Here's how the part is built. I have some questions about the finished solid (model axes, mm). Face numbers are marked on the shaded views. A direction names the side the tool comes from. Round coordinates to 2 decimals unless told otherwise and drop trailing zeros. Order: outer loops, then holes, each group sorted by start corner. A loop starts at its lowest first (then second) coordinate and runs counter-clockwise, first axis right, second up. Notation, with made-up numbers: (5.25, 36.5) - (45.25, 36.5) arc R32 ccw to (45.25, 63.5) - close; hole circle Ø8 at (13, 60). An arc over 180 degrees is marked (long way). Answer as a JSON object with one key per item and string values.
```python
from build123d import *

# Parameters (mm, degrees)
F0_R      = 14.5
F1_DEPTH  = 2
F2_R      = 11
F3_DEPTH  = 20
F4_R      = 2.075
F5_DEPTH  = 22.001
F6_W      = 3
F6_H      = 3.4
F7_DEPTH  = 2
F8_R      = 0.8
F9_R      = 0.5
F10_W     = 27.062299
F10_H     = 70.926305
F11_DEPTH = 22.001
F13_W     = 3.5
F13_H     = 9


with BuildPart() as f1:
    # F0 (on Top) → F1 (new body)
    with BuildSketch(Plane.XY):
        Circle(F0_R)
    extrude(amount=F1_DEPTH)

    # F2 (on face) → F3 (join)
    with BuildSketch(Plane.XY.offset(2)):
        Circle(F2_R)
    extrude(amount=F3_DEPTH)

    # F4 (on face) → F5 (cut, through all)
    with BuildSketch(Plane(origin=(0, 0, 0), x_dir=(1, 0, 0), z_dir=(0, 0, -1))):
        Circle(F4_R)
    extrude(amount=-F5_DEPTH, mode=Mode.SUBTRACT)

    # F6 (on face) → F7 (join)
    with BuildSketch(Plane.XY.offset(2)):
        with Locations((0, -11)):
            Rectangle(F6_W, F6_H)
    extrude(amount=F7_DEPTH)

    # F8
    f8_edges = [f1.edges().sort_by_distance(p)[0] for p in [
        (-1.5, -12.7, 3),
        (1.5, -12.7, 3),
    ]]
    fillet(f8_edges, radius=F8_R)

    # F9
    f9_edges = [f1.edges().sort_by_distance(p)[0] for p in [
        (-11, 0, 22),
    ]]
    fillet(f9_edges, radius=F9_R)

    # F10 (on Top) → F11 (cut, through all)
    with BuildSketch(Plane.XY):
        with Locations((13.531149, -0.320642)):
            Rectangle(F10_W, F10_H)
    extrude(amount=F11_DEPTH, mode=Mode.SUBTRACT)

    # F13 (on Front) → F14 (revolve, cut)
    with BuildSketch(Plane.XZ):
        with Locations((9.25, 13.5)):
            Rectangle(F13_W, F13_H)
    revolve(axis=Axis((0, 0, 13.307823), (0, 0, 1)), mode=Mode.SUBTRACT)


solid = f1.part
```
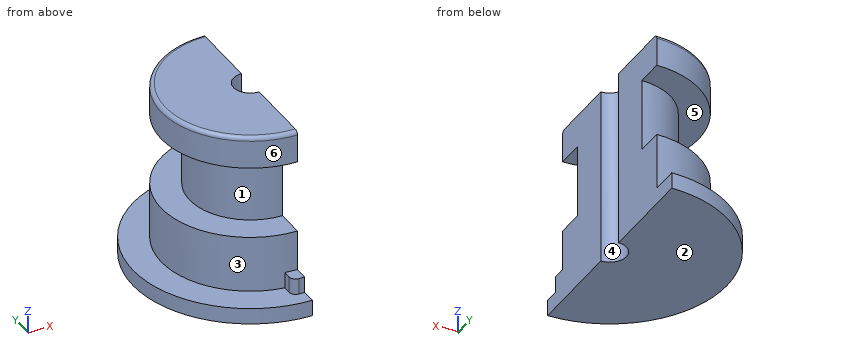
1. Thinking about a two-plate mould opening in Y: for the marked faces 4, 5 and 6, which applies, pulls with the +Y half, pulls with the -Y half, needs draft (parallel to the pull), parting line crosses it, or undercut?
Responses:
{"face 4": "undercut", "face 5": "needs draft", "face 6": "parting line crosses it"}
2. If I drill on L1, parallel to Z at x = -2.75, y = 9.5; L2, parallel to Z at x = -10.75, y = 9; L3, parallel to Y at x = -1.25, z = 13.5, over which ranges is the centre line in solid material (lowest first)? Write a range as [from, to].
Responses:
{"L1": "[0, 9], [18, 22]", "L2": "[0, 2]", "L3": "[-7.4, -1.66], [1.66, 7.4]"}
3. For P1, Ø8, axis at x = -4, y = 10.5, coming from the -Z side; P2, Ø0.5, axis at y = -11.5, z = 3.5, coming from the -X side; P3, Ø5, axis at x = -12.5, z = 13.5, coming from the -Y side; P4, Ø5, axis at x = -2, z = 8, coming from the +Y side, each with a flat end and sliding along its axis, tell me the tip position at first contact or that it passes through.
Responses:
{"P1": "z = 0", "P2": "x = -1.5", "P3": "through", "P4": "y = 11"}
4. Imagine slicing it at A-A (y = 0). List the corners of the cut face in (x, z) for me (3 decimals).
Responses:
{"outline": "(-14.5, 0) - (-2.075, 0) - (-2.075, 22) - (-10.5, 22) arc R0.5 ccw to (-11, 21.5) - (-11, 18) - (-7.5, 18) - (-7.5, 9) - (-11, 9) - (-11, 2) - (-14.5, 2) - close"}
5. For the marked faces 1, 2 and 3, which set-ups out of +Z, -Z, +X, -X, +Y, -Y let a thin tool reach every point of the face, with its end or its side?
Responses:
{"face 1": "-X", "face 2": "-Z, +X, -X, +Y, -Y", "face 3": "+Z, -X"}
6. Imagine slicing it at B-B (z = 4.75). List the corners of the cut face in (x, y) for me (3 decimals), plus the area to 3 significant figures.
Responses:
{"outline": "(0, -11) - (0, -2.075) arc R2.075 cw to (0, 2.075) - (0, 11) arc R11 ccw to start", "area": "183 mm2"}
7. Imagine slicing it at C-C (x = -13.5). List the corners of the cut face in (y, z) for me.
Responses:
{"outline": "(-5.29, 0) - (5.29, 0) - (5.29, 2) - (-5.29, 2) - close"}
